Input: part model. Units: mm. Frame: model coordinates. A direction names the side the tool comes from. Give positions to 0.01 mm unless a question says otherwise; leave off trailing zeros. Loops run counter-clockwise (first coordinate to the right, second up) from the corner with the lowest first, then second, coordinate; pieces in that order, holes last. Notation, with made-up numbers: (2, 36.5) - (56, 36.5) arc R20 ccw to (56, 62.5) - close; hole circle Ø5 at (83.25, -18). An arc over 180 degrees is marked (long way). Answer as a JSON object with one key per item and string values.
from build123d import *

# Parameters (mm, degrees)
SKETCH1_W                = 635
SKETCH1_H                = 711.2
SKETCH1_W_2              = 584.2
SKETCH1_H_2              = 660.4
BOSS_EXTRUDE2_DEPTH      = 50.8
SKETCH1_3_W              = 76.2
SKETCH1_3_H              = 76.2
BOSS_EXTRUDE3_DEPTH      = 101.6
BOSS_EXTRUDE3_DEPTH_BACK = 50.8
SKETCH3_W                = 863.6
SKETCH3_H                = 939.8
SKETCH3_W_2              = 635
SKETCH3_H_2              = 711.2
BOSS_EXTRUDE4_DEPTH      = 88.9
BOSS_EXTRUDE4_DEPTH_BACK = 25.4
FILLET1_R                = 50.8


with BuildPart() as part:
    # Sketch1 → Boss-Extrude2 (new body)
    with BuildSketch(Plane(origin=(0, 0, 0), x_dir=(1, 0, 0), z_dir=(0, 1, 0))):
        Rectangle(SKETCH1_W, SKETCH1_H)
        Rectangle(SKETCH1_W_2, SKETCH1_H_2, mode=Mode.SUBTRACT)
    extrude(amount=BOSS_EXTRUDE2_DEPTH)

    # Sketch1<3> → Boss-Extrude3 (add, two sides)
    with BuildSketch(Plane(origin=(0, 0, 0), x_dir=(1, 0, 0), z_dir=(0, 1, 0))) as boss_extrude3_sk:
        with Locations((-254, 292.1)):
            Rectangle(SKETCH1_3_W, SKETCH1_3_H)
        with Locations((254, 292.1)):
            Rectangle(SKETCH1_3_W, SKETCH1_3_H)
        with Locations((254, -292.1)):
            Rectangle(SKETCH1_3_W, SKETCH1_3_H)
        with Locations((-254, -292.1)):
            Rectangle(SKETCH1_3_W, SKETCH1_3_H)
    extrude(amount=BOSS_EXTRUDE3_DEPTH)
    extrude(boss_extrude3_sk.sketch, amount=-BOSS_EXTRUDE3_DEPTH_BACK)

    # Sketch3 → Boss-Extrude4 (add, two sides)
    with BuildSketch(Plane(origin=(0, 0, 0), x_dir=(1, 0, 0), z_dir=(0, 1, 0))) as boss_extrude4_sk:
        Rectangle(SKETCH3_W, SKETCH3_H)
        Rectangle(SKETCH3_W_2, SKETCH3_H_2, mode=Mode.SUBTRACT)
    extrude(amount=BOSS_EXTRUDE4_DEPTH)
    extrude(boss_extrude4_sk.sketch, amount=-BOSS_EXTRUDE4_DEPTH_BACK)

    # Fillet1
    fillet1_edges = [part.edges().sort_by_distance(p)[0] for p in [
        (-431.8, 31.75, 469.9),
        (-431.8, 31.75, -469.9),
        (431.8, 31.75, -469.9),
        (431.8, 31.75, 469.9),
    ]]
    fillet(fillet1_edges, radius=FILLET1_R)


solid = part.part
Item 1: Cut plane B-B (x = 15.5). Return loops of the section in (y, z).
Geometry check:
{"outline": "(-25.4, -469.9) - (88.9, -469.9) - (88.9, -355.6) - (50.8, -355.6) - (50.8, -330.2) - (0, -330.2) - (0, -355.6) - (-25.4, -355.6) - close; (-25.4, 355.6) - (0, 355.6) - (0, 330.2) - (50.8, 330.2) - (50.8, 355.6) - (88.9, 355.6) - (88.9, 469.9) - (-25.4, 469.9) - close"}
Item 2: Cut plane A-A (z = -303). Return loops of the section in (x, y), then the cut area to 3 significant figures.
Geometry check:
{"outline": "(-431.8, -25.4) - (-317.5, -25.4) - (-317.5, 0) - (-292.1, 0) - (-292.1, -50.8) - (-215.9, -50.8) - (-215.9, 101.6) - (-292.1, 101.6) - (-292.1, 50.8) - (-317.5, 50.8) - (-317.5, 88.9) - (-431.8, 88.9) - close; (215.9, -50.8) - (292.1, -50.8) - (292.1, 0) - (317.5, 0) - (317.5, -25.4) - (431.8, -25.4) - (431.8, 88.9) - (317.5, 88.9) - (317.5, 50.8) - (292.1, 50.8) - (292.1, 101.6) - (215.9, 101.6) - close", "area": "51,900 mm2"}
Item 3: Mould query, pull axis Z, two halves, no side actions, for faces 1 (the face through (215.9, 26, -292)), 2 (the face through (431.8, 33, 6)), 3 (the face through (417.314, 30.95, -454.624)). Classes: released by +Z, released by -Z, zero draft, split by the parting line, or undercut.
Geometry check:
{"face 1": "undercut", "face 2": "zero draft", "face 3": "released by -Z"}
Item 4: Cut plane C-C (y = 16.5). Return loops of the section in (x, z).
Geometry check:
{"outline": "(-431.8, -419.1) arc R50.8 ccw to (-381, -469.9) - (381, -469.9) arc R50.8 ccw to (431.8, -419.1) - (431.8, 419.1) arc R50.8 ccw to (381, 469.9) - (-381, 469.9) arc R50.8 ccw to (-431.8, 419.1) - close; hole (-292.1, -254) - (-215.9, -254) - (-215.9, -330.2) - (215.9, -330.2) - (215.9, -254) - (292.1, -254) - (292.1, 254) - (215.9, 254) - (215.9, 330.2) - (-215.9, 330.2) - (-215.9, 254) - (-292.1, 254) - close"}
Item 5: Contact query for a flat-ended pin moving along its axis: P1, Ø5, axis at x = 325, z = 106, coming from the -Y side. Output: stop coordinate, or through.
Geometry check:
{"P1": "stops at y = -25.4"}
Item 6: Material intervals for line 1 (X direction, y = 81.5, z = 279.5); line 2 (Z direction, x = -247.5, y = -0.5); line 3 (X direction, y = -43, z = 257.5), sorted ascending. Write a range as [from, to].
Geometry check:
{"line 1": "x = [-431.8, -317.5], [-292.1, -215.9], [215.9, 292.1], [317.5, 431.8]", "line 2": "z = [-469.9, -355.6], [-330.2, -254], [254, 330.2], [355.6, 469.9]", "line 3": "x = [-292.1, -215.9], [215.9, 292.1]"}
Item 7: Access query for faces 4 (the face through (253, -50.8, -293)), 5 (the face through (-292.1, -25, -292)), 6 (the face through (-4, 70, -355.6)), 7 (the face through (-215.9, 26, 293)). Directions: +Z, -Z, +X, -X, +Y, -Y. A direction counts if a zero-diameter tool reaches every point of the face in a straight line with its end or side. Return the directions, or none.
Geometry check:
{"face 4": "+Z, -Z, +X, -X, -Y", "face 5": "-Y", "face 6": "+Y", "face 7": "+Y, -Y"}
Item 8: Cut plane D-D (x = 242). Return loops of the section in (y, z).
Geometry check:
{"outline": "(-50.8, -330.2) - (0, -330.2) - (0, -355.6) - (-25.4, -355.6) - (-25.4, -469.9) - (88.9, -469.9) - (88.9, -355.6) - (50.8, -355.6) - (50.8, -330.2) - (101.6, -330.2) - (101.6, -254) - (-50.8, -254) - close; (-50.8, 254) - (101.6, 254) - (101.6, 330.2) - (50.8, 330.2) - (50.8, 355.6) - (88.9, 355.6) - (88.9, 469.9) - (-25.4, 469.9) - (-25.4, 355.6) - (0, 355.6) - (0, 330.2) - (-50.8, 330.2) - close"}
